CAD build for the part. Positions are in the model's coordinates, mm. Give positions to 0.01 mm unless a question says otherwise; leave off trailing zeros. Order: outer loops, then holes, each group sorted by start corner. A loop starts at its lowest first (then second) coordinate and runs counter-clockwise, first axis right, second up.
Item 1: Band-saw the part on C-C on y = -6.5. Give the cut face in (x, z), plus the area to 3 significant figures.
Item 2: Band-saw the part on A-A on x = 0. Give the cut face in (y, z).
Item 3: Flat gauge pins, fed straight in: P1, Ø2, axis at x = 6, y = -1, coming from the +Z side; P2, Ø3, axis at x = 0.5, z = 39.5, coming from the +Y side. Where does each tip first touch, or does it go through?
Item 4: Wall check: L1, parallel to Y at x = -4.5, z = 59; L2, parallel to Y at x = -6, z = 5; L3, parallel to Y at x = -3.25, z = 62. Give the ranges that are in metal, low to high.
```python
from build123d import *

# Parameters (mm, degrees)
SKETCH1_R           = 2.5
BOSS_EXTRUDE1_DEPTH = 70


with BuildPart() as part:
    # Sketch1 → Boss-Extrude1 (new body)
    with BuildSketch(Plane.XY):
        with BuildLine():
            Line((-9.707106781, -3.2), (-8.6, -3.2))
            Line((-8.6, -3.2), (-8.6, -7.185786438))
            Line((-8.6, -7.185786438), (-3.445719569, -2.031506006))
            ThreePointArc((-3.445719569, -2.031506006), (-4, 0), (-3.445719569, 2.031506006))
            Line((-3.445719569, 2.031506006), (-8.6, 7.185786438))
            Line((-8.6, 7.185786438), (-8.6, 3.2))
            Line((-8.6, 3.2), (-9.707106781, 3.2))
            Line((-9.707106781, 3.2), (-9.707106781, 3.877544562))
            Line((-9.707106781, 3.877544562), (-10, 3.877544562))
            Line((-10, 3.877544562), (-10, 9))
            ThreePointArc((-10, 9), (-9.707106781, 9.707106781), (-9, 10))
            Line((-9, 10), (-3.877544562, 10))
            Line((-3.877544562, 10), (-3.877544562, 9.707106781))
            Line((-3.877544562, 9.707106781), (-3.2, 9.707106781))
            Line((-3.2, 9.707106781), (-3.2, 8.6))
            Line((-3.2, 8.6), (-7.185786438, 8.6))
            Line((-7.185786438, 8.6), (-2.031506006, 3.445719569))
            ThreePointArc((-2.031506006, 3.445719569), (0, 4), (2.031506006, 3.445719569))
            Line((2.031506006, 3.445719569), (7.185786438, 8.6))
            Line((7.185786438, 8.6), (3.2, 8.6))
            Line((3.2, 8.6), (3.2, 9.707106781))
            Line((3.2, 9.707106781), (3.877544562, 9.707106781))
            Line((3.877544562, 9.707106781), (3.877544562, 10))
            Line((3.877544562, 10), (9, 10))
            ThreePointArc((9, 10), (9.707106781, 9.707106781), (10, 9))
            Line((10, 9), (10, 3.877544562))
            Line((10, 3.877544562), (9.707106781, 3.877544562))
            Line((9.707106781, 3.877544562), (9.707106781, 3.2))
            Line((9.707106781, 3.2), (8.6, 3.2))
            Line((8.6, 3.2), (8.6, 7.185786438))
            Line((8.6, 7.185786438), (3.445719569, 2.031506006))
            ThreePointArc((3.445719569, 2.031506006), (4, 0), (3.445719569, -2.031506006))
            Line((3.445719569, -2.031506006), (8.6, -7.185786438))
            Line((8.6, -7.185786438), (8.6, -3.2))
            Line((8.6, -3.2), (9.707106781, -3.2))
            Line((9.707106781, -3.2), (9.707106781, -3.877544562))
            Line((9.707106781, -3.877544562), (10, -3.877544562))
            Line((10, -3.877544562), (10, -9))
            ThreePointArc((10, -9), (9.707106781, -9.707106781), (9, -10))
            Line((9, -10), (3.877544562, -10))
            Line((3.877544562, -10), (3.877544562, -9.707106781))
            Line((3.877544562, -9.707106781), (3.2, -9.707106781))
            Line((3.2, -9.707106781), (3.2, -8.6))
            Line((3.2, -8.6), (7.185786438, -8.6))
            Line((7.185786438, -8.6), (2.031506006, -3.445719569))
            ThreePointArc((2.031506006, -3.445719569), (0, -4), (-2.031506006, -3.445719569))
            Line((-2.031506006, -3.445719569), (-7.185786438, -8.6))
            Line((-7.185786438, -8.6), (-3.2, -8.6))
            Line((-3.2, -8.6), (-3.2, -9.707106781))
            Line((-3.2, -9.707106781), (-3.877544562, -9.707106781))
            Line((-3.877544562, -9.707106781), (-3.877544562, -10))
            Line((-3.877544562, -10), (-9, -10))
            ThreePointArc((-9, -10), (-9.707106781, -9.707106781), (-10, -9))
            Line((-10, -9), (-10, -3.877544562))
            Line((-10, -3.877544562), (-9.707106781, -3.877544562))
            Line((-9.707106781, -3.877544562), (-9.707106781, -3.2))
        make_face()
        Circle(SKETCH1_R, mode=Mode.SUBTRACT)
    extrude(amount=BOSS_EXTRUDE1_DEPTH)


solid = part.part
```
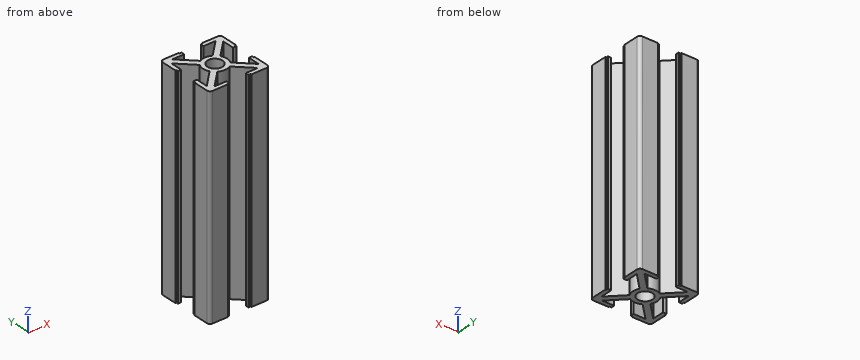
The answers:
1. outline: (-10, 0) - (-8.6, 0) - (-8.6, 70) - (-10, 70) - close; (-7.91, 0) - (-5.09, 0) - (-5.09, 70) - (-7.91, 70) - close; (5.09, 0) - (7.91, 0) - (7.91, 70) - (5.09, 70) - close; (8.6, 0) - (10, 0) - (10, 70) - (8.6, 70) - close
1. area: 592 mm2
2. outline: (-4, 0) - (-2.5, 0) - (-2.5, 70) - (-4, 70) - close; (2.5, 0) - (4, 0) - (4, 70) - (2.5, 70) - close
3. P1: passes through
3. P2: stops at y = 4
4. L1: y = -10 to -8.6, -5.91 to -3.09, 3.09 to 5.91, 8.6 to 10
4. L2: y = -10 to -8.6, -7.41 to -4.59, 4.59 to 7.41, 8.6 to 10
4. L3: y = -9.71 to -8.6, -4.66 to 4.66, 8.6 to 9.71
